For this review, take the finished solid that the model builds, in its own axes (mm). Coordinates: 2 decimals unless noted, no trailing zeros. Write each loop counter-clockwise with the first axis right and the second up, starting at its lowest first coordinate (ties: lowest second). Pieces come first, ordered by that corner, then holes.
1) Mouldability with a two-part tool opening along Y and no side actions: class faces 1 (the face through (-0.193, 6.147, -0.345)), 2 (the face through (3.33, 3.14, -0.35)), 3 (the face through (-3.28, 3.19, -0.35)), 4 (the face through (0.1, 3.4, 0)) as pulls with the +Y half, pulls with the -Y half, needs draft (parallel to the pull), parting line crosses it, or undercut.
2) We need section D-D on y = 5. Write out the cut boundary in (x, z).
3) To check wall thickness, follow line 1 along X through (y, z) = (3.25, -0.05); line 2 along X through (y, z) = (3.75, -0.5); line 3 along X through (y, z) = (-3.5, -0.1). State the ranges of each line that lie inside material, in increasing order.
4) We need section C-C on x = -1.25. Write out the cut boundary in (y, z).
5) Insertion check: P1, Ø1.5, axis at x = -3, y = 4.5, coming from the +Z side. The pin has a flat end and moves straight along its axis. Give the tip position at first contact, or say it passes through.
6) We need section A-A on y = 0. Write out the cut boundary in (x, z).
from build123d import *

# Parameters (mm, degrees)
BODY_DEPTH = 0.7


with BuildPart() as part:
    # BodySke → Body (new body)
    with BuildSketch(Plane.XY):
        with BuildLine():
            Line((2.954423259, 0.520944533), (4.099428621, 0.722839871))
            ThreePointArc((4.099428621, 0.722839871), (4.363883059, 0.900217065), (4.410660695, 1.215194321))
            ThreePointArc((4.410660695, 1.215194321), (3.304815126, 3.16367223), (1.406428042, 4.353456691))
            ThreePointArc((1.406428042, 4.353456691), (1.089710164, 4.320462692), (0.900966453, 4.063997041))
            Line((0.900966453, 4.063997041), (0.80903451, 3.649318842))
            ThreePointArc((0.80903451, 3.649318842), (0, 3), (-0.80903451, 3.649318842))
            Line((-0.80903451, 3.649318842), (-0.900966453, 4.063997041))
            ThreePointArc((-0.900966453, 4.063997041), (-1.089710164, 4.320462692), (-1.406428042, 4.353456691))
            ThreePointArc((-1.406428042, 4.353456691), (-3.304815126, 3.16367223), (-4.410660695, 1.215194321))
            ThreePointArc((-4.410660695, 1.215194321), (-4.363883059, 0.900217065), (-4.099428621, 0.722839871))
            Line((-4.099428621, 0.722839871), (-2.954423259, 0.520944533))
            ThreePointArc((-2.954423259, 0.520944533), (-2.974334584, -0.391578577), (-2.718923361, -1.267854785))
            Line((-2.718923361, -1.267854785), (-3.446179756, -3.574417389))
            ThreePointArc((-3.446179756, -3.574417389), (-4.053778864, -4.111935463), (-4.813608561, -3.827750334))
            ThreePointArc((-4.813608561, -3.827750334), (0, 6.15), (4.813608561, -3.827750334))
            ThreePointArc((4.813608561, -3.827750334), (4.053778864, -4.111935463), (3.446179756, -3.574417389))
            Line((3.446179756, -3.574417389), (2.718923361, -1.267854785))
            ThreePointArc((2.718923361, -1.267854785), (2.974334584, -0.391578577), (2.954423259, 0.520944533))
        make_face()
    extrude(amount=-BODY_DEPTH)


solid = part.part
Result:
1. face 1: parting line crosses it
1. face 2: undercut
1. face 3: undercut
1. face 4: needs draft
2. outline: (-3.58, -0.7) - (3.58, -0.7) - (3.58, 0) - (-3.58, 0) - close
3. line 1: x = -5.22 to -3.22, -0.59 to 0.59, 3.22 to 5.22
3. line 2: x = -4.87 to -2.62, -0.83 to 0.83, 2.62 to 4.87
3. line 3: x = -5.06 to -3.42, 3.42 to 5.06
4. outline: (4.37, -0.7) - (6.02, -0.7) - (6.02, 0) - (4.37, 0) - close
5. P1: stops at z = 0
6. outline: (-6.15, -0.7) - (-3, -0.7) - (-3, 0) - (-6.15, 0) - close; (3, -0.7) - (6.15, -0.7) - (6.15, 0) - (3, 0) - close
